Can you work these out from the model? Positions are in its coordinate system, mm. A direction names the side the tool comes from. Give positions to 0.01 mm unless a question says otherwise; leave off trailing zeros. Write each loop counter-clockwise with the first axis right and the second up, starting at its lowest first coordinate (ties: lowest second). Pieces come first, ordered by that corner, then holes. Notation, with made-up numbers: (48.25, 66) -> (60.25, 66) arc R8 ccw to (60.25, 80) -> close; hole circle Ø7 at (20, -31.5). An arc over 180 degrees is marked (long way). One line per item, written item: value.
Autodesk Inventor part; units mm, degrees
ref_plane "YZ Plane" through (0, 0, 0) normal (1, 0, 0) x (0, 1, 0)
ref_plane "XZ Plane" through (0, 0, 0) normal (0, 1, 0) x (-1, 0, 0)
ref_plane "XY Plane" through (0, 0, 0) normal (0, 0, 1) x (1, 0, 0)
sketch "Sketch1" plane through (0, 0, 0) normal (0, 1, 0) x (-1, 0, 0)
  line L0 (0, 0) -> (-86, 0)
  line L1 (-86, 0) -> (-86, -169)
  line L2 (-86, -169) -> (0, -169)
  line L3 (0, -169) -> (0, 0)
  circle A0 centre (-12.7, -25.4) radius 3.175
  circle A1 centre (-12.7, -127) radius 3.175
  circle A2 centre (-76.2, -25.4) radius 3.175
  circle A3 centre (-76.2, -127) radius 3.175
  line L4 (0, -169) -> (-86, -169)
  line L5 (-86, -169) -> (-86, -165.825)
  line L6 (-86, -165.825) -> (0, -165.825)
  line L7 (0, -165.825) -> (0, -169)
  point P0 (0, -165.825)
  dimension "d0" = 6.35
  dimension "d1" = 169
  dimension "d2" = 86
  dimension "d3" = 12.7
  dimension "d4" = 25.4
  dimension "d7" = 101.6
  dimension "d10" = 63.5
  dimension "d31" = 3.175
extrude "Extrusion1" add sketch "Sketch1" along normal blind 3.175 contours L3 L6 L1 L0
sketch "Sketch3" plane through (0, 3.175, 0) normal (0, 1, 0) x (1, 0, 0)
  line L0 (0, 0) -> (86, 0)
  line L1 (21.875, 0) -> (64.125, 0)
  line L2 (64.125, 0) -> (64.125, 165.825)
  line L3 (64.125, 165.825) -> (21.875, 165.825)
  line L4 (21.875, 165.825) -> (21.875, 0)
  line L5 (0, 165.825) -> (0, 0)
  line L6 (86, 0) -> (86, 165.825)
  line L7 (43, 0) -> (43.307, 154.432) construction
  line L8 (86.614, 154.432) -> (0, 154.432) construction
  line L9 (43, 0) -> (43, 165.825) construction
  line L10 (86, 165.825) -> (0, 165.825)
  point P0 (64.125, 0)
  dimension "d28" = 42.25
extrude "Extrusion3" add sketch "Sketch3" along normal blind 12.192 contours L4 L3 L2 L0
extrude "Extrusion4" add sketch "Sketch1" along normal blind 101.981 contours L3 L2 L1 L6
sketch "Sketch4" plane through (86, 0, -169) normal (0, 0, -1) x (-1, 0, 0)
  circle A0 centre (43.3338, 58.6472) radius 38.1
  circle A1 centre (8.5085, 93.4725) radius 3.4925
  line L0 (0, 0) -> (0, 101.981)
  line L1 (0, 101.981) -> (86, 101.981)
  circle A2 centre (78.1055, 93.4725) radius 3.4925
  circle A3 centre (8.5085, 23.8755) radius 3.4925
  circle A4 centre (78.1055, 23.8755) radius 3.4925
  point P0 (86, 0)
  dimension "d34" = 76.2
  dimension "d35" = 6.985
  dimension "d36" = 8.5085
  dimension "d38" = 8.5085
  dimension "d41" = 69.597
  dimension "d44" = 69.597
  dimension "d47" = 43.3338
  dimension "d48" = 43.3338
extrude "Extrusion5" cut sketch "Sketch4" against normal through all
fillet "Fillet1" radius 12.7 2 edges at (75.0625, 3.175, -165.825) (10.9375, 3.175, -165.825)
fillet "Fillet2" radius 6.35 2 edges at (86, 101.981, -167.4125) (0, 101.981, -167.4125)
equation "\"d28\" = 0.25 * d1"
properties part number "MotorStandoff"
1) We'd pull the mould along X, two halves only. Please class faces 1 (the face through (1.91, 100.17, -167.39)), 2 (the face through (84.09, 100.17, -167.43)), 3 (the face through (13.11, 1.57, -28.55)): released by +X, released by -X, zero draft, split by the parting line, or undercut.
Answer list:
face 1: released by -X
face 2: released by +X
face 3: undercut
2) Will these pins go through, and if not, where does the flat tip stop? pin 1 (10 mm diameter, centred on y = 17, z = -19.5, fed in from +X) (3 decimals); pin 2 (11 mm diameter, centred on x = 9.5, z = -92, fed in from +Y) (3 decimals); pin 3 (9 mm diameter, centred on x = 77.49, y = 23.88, fed in from +Z) (3 decimals).
Answer list:
pin 1: stops at x = 64.125
pin 2: stops at y = 3.175
pin 3: stops at z = -165.825
3) I need wall thicknesses on L1, parallel to Z at x = 76, y = 2; L2, parallel to Y at x = 42, z = -134; L3, parallel to Y at x = 66, z = -65.5 (3 decimals). Which ranges of each line are inside material? Lowest first, please.
Answer list:
L1: z = -169 to -130.17, -123.83 to -28.57, -22.23 to 0
L2: y = 0 to 15.37
L3: y = 0 to 3.175
4) If we section it at B-B (z = -25.4): Write out the boundary of the cut face in (x, y) (3 decimals), and give its area (3 significant figures).
Answer list:
outline: (0, 0) -> (9.525, 0) -> (9.525, 3.175) -> (0, 3.175) -> close; (15.875, 0) -> (73.025, 0) -> (73.025, 3.175) -> (64.125, 3.175) -> (64.125, 15.367) -> (21.875, 15.367) -> (21.875, 3.175) -> (15.875, 3.175) -> close; (79.375, 0) -> (86, 0) -> (86, 3.175) -> (79.375, 3.175) -> close
area: 748 mm^2
5) If we section it at C-C (x = 76.2): Write out the boundary of the cut face in (y, z) (3 decimals).
Answer list:
outline: (0, -169) -> (20.631, -169) -> (20.631, -165.825) -> (15.875, -165.825) arc R12.7 cw to (3.175, -153.125) -> (3.175, -130.175) -> (0, -130.175) -> close; (0, -123.825) -> (3.175, -123.825) -> (3.175, -28.575) -> (0, -28.575) -> close; (0, -22.225) -> (3.175, -22.225) -> (3.175, 0) -> (0, 0) -> close; (27.12, -169) -> (40.561, -169) -> (40.561, -165.825) -> (27.12, -165.825) -> close; (76.733, -169) -> (90.228, -169) -> (90.228, -165.825) -> (76.733, -165.825) -> close; (96.717, -169) -> (101.981, -169) -> (101.981, -165.825) -> (96.717, -165.825) -> close
6) For faces 4 (the face through (82, 58, -165.825)), 5 (the face through (11, 3.175, -75)), 6 (the face through (75, 3.175, -75)), which set-ups out of +Z, -Z, +X, -X, +Y, -Y let a thin tool reach every point of the face, with its end or its side?
Answer list:
face 4: +Z, +X, -X, +Y
face 5: +Z, -X, +Y
face 6: +Z, +X, +Y
7) If we section it at A-A (y = 80): Write out the boundary of the cut face in (x, z) (3 decimals).
Answer list:
outline: (0, -169) -> (11.112, -169) -> (11.112, -165.825) -> (0, -165.825) -> close; (74.22, -169) -> (86, -169) -> (86, -165.825) -> (74.22, -165.825) -> close
8) If we section it at D-D (x = 13.5): Write out the boundary of the cut face in (y, z) (3 decimals).
Answer list:
outline: (0, -169) -> (34.133, -169) -> (34.133, -165.825) -> (15.875, -165.825) arc R12.7 cw to (3.175, -153.125) -> (3.175, -130.073) -> (0, -130.073) -> close; (0, -123.927) -> (3.175, -123.927) -> (3.175, -28.473) -> (0, -28.473) -> close; (0, -22.327) -> (3.175, -22.327) -> (3.175, 0) -> (0, 0) -> close; (83.161, -169) -> (101.981, -169) -> (101.981, -165.825) -> (83.161, -165.825) -> close
